from build123d import *

# Parameters (mm, degrees)
SKETCH1_W          = 82.55
SKETCH1_H          = 82.55
SKETCH1_R          = 34.1503
EXTRUDE1_DEPTH     = 15.875
CUT_EXTRUDE1_DEPTH = 8.7376
HOLE1_D            = 8.7122
HOLE1_DEPTH        = 7.1374


with BuildPart() as part:
    # Sketch1 → Extrude1 (new body)
    with BuildSketch(Plane(origin=(0, 0, 0), x_dir=(1, 0, 0), z_dir=(0, 1, 0))):
        Rectangle(SKETCH1_W, SKETCH1_H)
        with Locations(Location((0, 0, 0), (0, 0, 270))):  # turned: the seam where the file's is
            Circle(SKETCH1_R, mode=Mode.SUBTRACT)
    extrude(amount=EXTRUDE1_DEPTH)

    # Sketch2 → Cut-Extrude1 (cut)
    with BuildSketch(Plane(origin=(0, 15.875, 0), x_dir=(1, 0, 0), z_dir=(0, 1, 0))):
        with BuildLine():
            Line((23.853264661, -41.275), (41.275, -41.275))
            Line((41.275, -41.275), (41.275, -23.853264661))
            ThreePointArc((41.275, -23.853264661), (25.766943879, -25.766943879), (23.853264661, -41.275))
        make_face()
        with BuildLine():
            Line((41.275, 41.275), (41.275, 23.853264661))
            ThreePointArc((41.275, 23.853264661), (25.766943879, 25.766943879), (23.853264661, 41.275))
            Line((23.853264661, 41.275), (41.275, 41.275))
        make_face()
        with BuildLine():
            Line((-23.853264661, 41.275), (-41.275, 41.275))
            Line((-41.275, 41.275), (-41.275, 23.853264661))
            ThreePointArc((-41.275, 23.853264661), (-25.766943879, 25.766943879), (-23.853264661, 41.275))
        make_face()
        with BuildLine():
            Line((-41.275, -41.275), (-41.275, -23.853264661))
            ThreePointArc((-41.275, -23.853264661), (-25.766943879, -25.766943879), (-23.853264661, -41.275))
            Line((-23.853264661, -41.275), (-41.275, -41.275))
        make_face()
    extrude(amount=-CUT_EXTRUDE1_DEPTH, mode=Mode.SUBTRACT)

    # Hole1
    with Locations(Plane(origin=(0, 7.1374, 0), x_dir=(-1, 0, 0), z_dir=(0, 1, 0))):
        with Locations((31.75, 31.75), (31.75, -31.75), (-31.75, 31.75), (-31.75, -31.75)):
            Hole(HOLE1_D / 2, depth=HOLE1_DEPTH)

    # Sketch5 → Cut-Revolve1 (revolve, cut)
    with BuildSketch(Plane(origin=(0, 0, 0), x_dir=(0, 0, -1), z_dir=(1, 0, 0)), mode=Mode.PRIVATE) as cut_revolve1_sk:
        Polygon((-35.306, 15.875), (-34.1503, 15.875), (-34.1503, 14.7193), align=None)
        Polygon((-34.1503, 1.1557), (-35.306, 0), (-34.1503, 0), align=None)
    revolve(cut_revolve1_sk.sketch.rotate(Axis((0, 0, 0), (0, 1, 0)), 180), axis=Axis((0, 0, 0), (0, 1, 0)), mode=Mode.SUBTRACT)  # turned: the seam where the file's is


solid = part.part
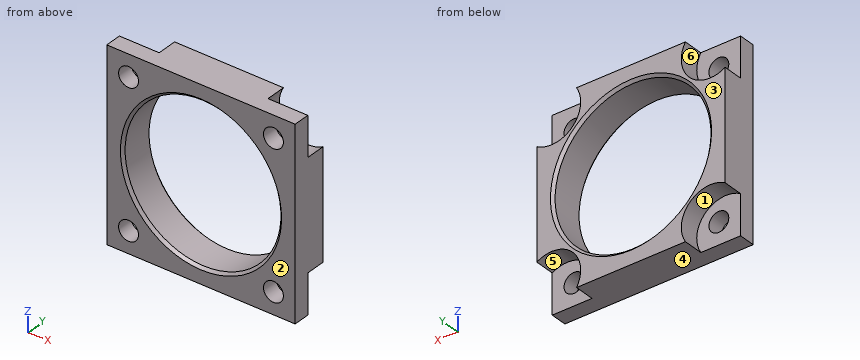
For this review, take the finished solid that the model builds, in its own axes (mm). Face numbers are marked on the shaded views. A direction names the side the tool comes from. Round coordinates to 2 decimals unless told otherwise and drop trailing zeros. Loops run counter-clockwise (first coordinate to the right, second up) from the corner with the lowest first, then second, coordinate; pieces in that order, holes last. Notation, with made-up numbers: (45.25, 40.5) - (83.25, 40.5) arc R26 ccw to (83.25, 61.5) - close; hole circle Ø11 at (85, 36). An arc over 180 degrees is marked (long way). One line per item, written item: value. Start each with the question number.
Item 1: The part is to be moulded in two halves that separate along Z. For the marked faces 3, 4, 5 and 6, say which applies: +Z half, -Z half, draft (parallel to the pull), parting line (faces both ways), or undercut.
Item 2: Clearance check with flat-ended pins moving along their axes: pin 1 Ø9.5 at (x, z) = (-35, 36) entering from +Y; pin 2 Ø6 at (y, z) = (10.5, -27.5) entering from +X. State where each tip first meets the part, or that it passes through.
Item 3: Take a section at A-A (z = 0). Give the boundary of the cut face in (x, y) (3 decimals).
Item 4: Take a section at B-B (y = 4.75). Give the boundary of the cut face in (x, z) (3 decimals), plus the area to 3 significant figures.
Item 5: Take a section at C-C (x = 0). Give the boundary of the cut face in (y, z) (3 decimals), plus the area to 3 significant figures.
Item 6: For L1, parallel to Z at x = 31.75, y = 3.25 (3 decimals); L2, parallel to X at y = 4, z = 0 (3 decimals); L3, parallel to X at y = 5.75, z = -30 (3 decimals), list the stretches that pass through material, from the lowest coordinate up.
Item 7: Take a section at D-D (y = 12.75). Give the boundary of the cut face in (x, z) (3 decimals), plus the area to 3 significant figures.
Item 8: For the marked faces 1 and 2, list the 3-axis set-ups (+Z, -Z, +X, -X, +Y, -Y) from which the entire face can be reached by the end or side of a thin tool; tool diameter is ignored.
Answer below:
1. face 3: draft
1. face 4: -Z half
1. face 5: undercut
1. face 6: undercut
2. pin 1: stops at y = 7.14
2. pin 2: stops at x = 27.24
3. outline: (-41.275, 0) - (-35.306, 0) - (-34.15, 1.156) - (-34.15, 14.719) - (-35.306, 15.875) - (-41.275, 15.875) - close; (34.15, 1.156) - (35.306, 0) - (41.275, 0) - (41.275, 15.875) - (35.306, 15.875) - (34.15, 14.719) - close
4. outline: (-41.275, -41.275) - (41.275, -41.275) - (41.275, 41.275) - (-41.275, 41.275) - close; hole circle Ø8.712 at (-31.75, -31.75); hole circle Ø8.712 at (-31.75, 31.75); hole circle Ø68.301 at (0, 0); hole circle Ø8.712 at (31.75, -31.75); hole circle Ø8.712 at (31.75, 31.75)
4. area: 2,910 mm2
5. outline: (0, -41.275) - (15.875, -41.275) - (15.875, -35.306) - (14.719, -34.15) - (1.156, -34.15) - (0, -35.306) - close; (0, 35.306) - (1.156, 34.15) - (14.719, 34.15) - (15.875, 35.306) - (15.875, 41.275) - (0, 41.275) - close
5. area: 224 mm2
6. L1: z = -41.275 to -36.106, -27.394 to -12.577, 12.577 to 27.394, 36.106 to 41.275
6. L2: x = -41.275 to -34.15, 34.15 to 41.275
6. L3: x = -41.275 to -35.739, -27.761 to -16.317, 16.317 to 27.761, 35.739 to 41.275
7. outline: (-41.275, -23.853) arc R12.7 cw to (-23.853, -41.275) - (23.853, -41.275) arc R12.7 cw to (41.275, -23.853) - (41.275, 23.853) arc R12.7 cw to (23.853, 41.275) - (-23.853, 41.275) arc R12.7 cw to (-41.275, 23.853) - close; hole circle Ø68.301 at (0, 0)
7. area: 1,840 mm2
8. face 1: +Y
8. face 2: +Z, -Z, +X, -X, -Y
